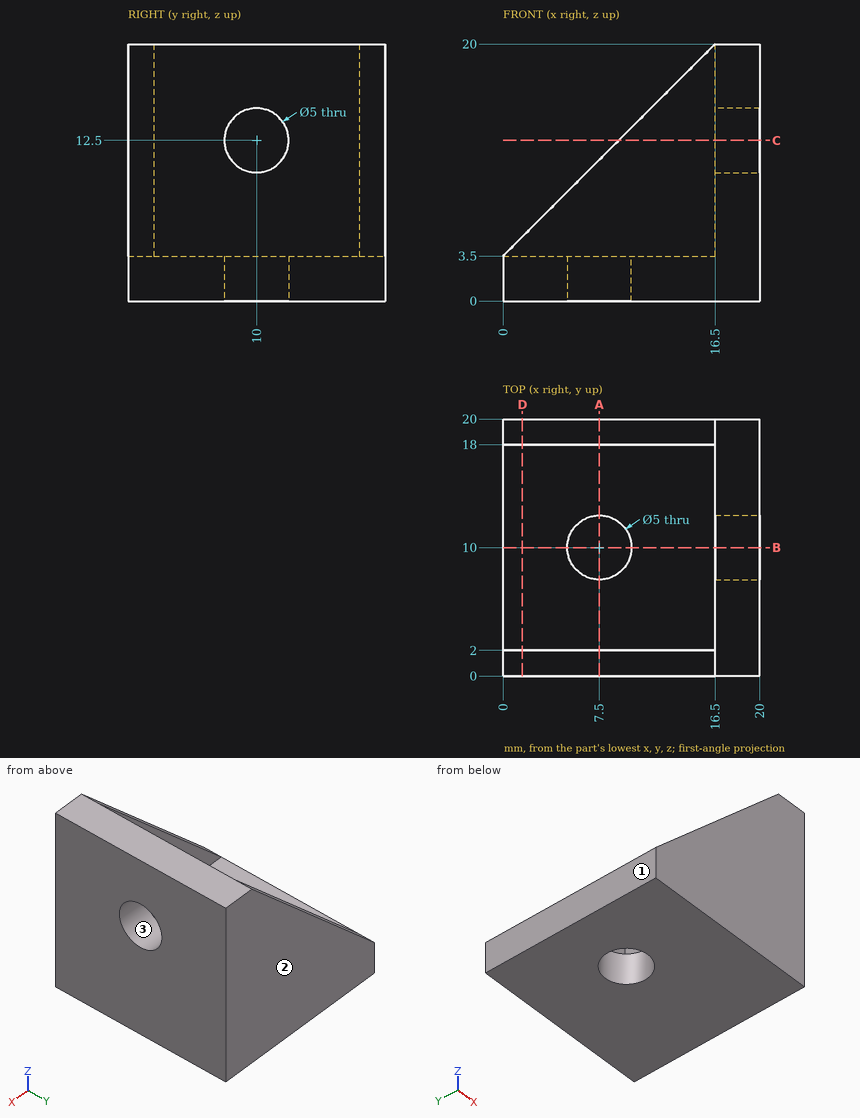
Study the drawing (mm; zero at the part's minimum x, y, z) and answer. Coordinates: 2 decimals unless noted, no trailing zeros. Loops run counter-clockwise (first coordinate to the right, second up) from the corner with the lowest first, then second, coordinate; pieces in that order, holes last. Notation, with made-up numbers: M 1.25,84 L 19.25,84 A23 ccw 19.25,114 Z; hole C -24,-32.5 d5. An arc over 180 degrees is marked long. Answer as a JSON object with one key per item and string values. Group by question number.
Item 1: Consider L1, parallel to Y at x = 19.25, z = 12.5; L2, parallel to Y at x = 12, z = 11.75; L3, parallel to Z at x = 10.75, y = 3. Determine where each line is inside the solid, lowest interval first.
Item 2: Each of these flat-tipped pins is pushed along its axis until it touches: P1, Ø4, axis at x = 5.5, z = 14, coming from the +Y side; P2, Ø8, axis at y = 6.5, z = 9, coming from the -X side. Where does it stop, or does it pass through?
Item 3: Section C-C (z = 12.5) is taken. Write down the section's boundary in (x, y).
Item 4: Section A-A (x = 7.5) is taken. Write down the section's boundary in (y, z), and give its area (3 significant figures).
Item 5: Section D-D (x = 1.5) is taken. Write down the section's boundary in (y, z), and give its area (3 significant figures).
Item 6: Determine the mould class of the marked faces 1, 2 and 3 for opening direction Y: +Y half, -Y half, draft (parallel to the pull), parting line (faces both ways), or undercut.
Item 7: Section B-B (y = 10) is taken. Write down the section's boundary in (x, z), and give its area (4 significant figures).
Solved:
{
 "1": {"L1": "y = 0 to 7.5, 12.5 to 20", "L2": "y = 0 to 2, 18 to 20", "L3": "z = 0 to 3.5"},
 "2": {"P1": "passes through", "P2": "stops at x = 16.5"},
 "3": {"outline": "M 9,0 L 20,0 L 20,7.5 L 16.5,7.5 L 16.5,2 L 9,2 Z; M 9,18 L 16.5,18 L 16.5,12.5 L 20,12.5 L 20,20 L 9,20 Z"},
 "4": {"outline": "M 0,0 L 7.5,0 L 7.5,3.5 L 2,3.5 L 2,11 L 0,11 Z; M 12.5,0 L 20,0 L 20,11 L 18,11 L 18,3.5 L 12.5,3.5 Z", "area": "82.5 mm2"},
 "5": {"outline": "M 0,0 L 20,0 L 20,5 L 18,5 L 18,3.5 L 2,3.5 L 2,5 L 0,5 Z", "area": "76.0 mm2"},
 "6": {"face 1": "draft", "face 2": "+Y half", "face 3": "undercut"},
 "7": {"outline": "M 0,0 L 5,0 L 5,3.5 L 0,3.5 Z; M 10,0 L 20,0 L 20,10 L 16.5,10 L 16.5,3.5 L 10,3.5 Z; M 16.5,15 L 20,15 L 20,20 L 16.5,20 Z", "area": "92.75 mm2"}
}
